from build123d import *

# Parameters (mm, degrees)
BOSS_EXTRUDE1_DEPTH = 2
SKETCH2_R           = 6
CUT_EXTRUDE1_DEPTH  = 124
BOSS_EXTRUDE2_DEPTH = 20


with BuildPart() as part:
    # Sketch1 → Boss-Extrude1 (new body)
    with BuildSketch(Plane.XY):
        Polygon((-55, 0), (55, 0), (20, 110), (-20, 110), align=None)
    extrude(amount=BOSS_EXTRUDE1_DEPTH)

    # Sketch2 → Cut-Extrude1 (cut, through all)
    with BuildSketch(Plane.XY.offset(2)):
        with Locations((0, 90)):
            Circle(SKETCH2_R)
    extrude(amount=-CUT_EXTRUDE1_DEPTH, mode=Mode.SUBTRACT)

    # Sketch4 → Boss-Extrude2 (add)
    with BuildSketch(Plane.XY.offset(2)):
        Polygon((-55, 0), (-54.363636364, 2), (54.363636364, 2), (55, 0), align=None)
    extrude(amount=BOSS_EXTRUDE2_DEPTH)


solid = part.part
Here's how the part is built. I have some questions about the finished solid (model axes, mm). Coordinates: 2 decimals unless noted, no trailing zeros. Order: outer loops, then holes, each group sorted by start corner. A loop starts at its lowest first (then second) coordinate and runs counter-clockwise, first axis right, second up. Notation, with made-up numbers: (0, -39) -> (56, -39) arc R12 ccw to (56, -16) -> close; hole circle Ø10 at (11, -22). An arc over 180 degrees is marked (long way). Answer in a Markdown table with one row per item.
(1) I want a section at B-B on y = 93. List the corners of the cut face in (x, z) for me.
Answer key:
| item | result |
|---|---|
| outline | (-25.41, 0) -> (-5.2, 0) -> (-5.2, 2) -> (-25.41, 2) -> close; (5.2, 0) -> (25.41, 0) -> (25.41, 2) -> (5.2, 2) -> close |
(2) Will these pins go through, and if not, where does the flat tip stop? pin 1 Ø12 at (y, z) = (43.5, 5) entering from +X; pin 2 Ø4 at (x, z) = (18.5, 13) entering from +Y; pin 3 Ø10 at (x, y) = (-38, 61.5) entering from -Z; pin 4 Ø10 at (x, y) = (-18, 48) entering from +Z.
Answer key:
| item | result |
|---|---|
| pin 1 | x = 42.81 |
| pin 2 | y = 2 |
| pin 3 | z = 0 |
| pin 4 | z = 2 |
(3) I want a section at D-D on x = -33. List the corners of the cut face in (y, z) for me.
Answer key:
| item | result |
|---|---|
| outline | (0, 0) -> (69.14, 0) -> (69.14, 2) -> (2, 2) -> (2, 22) -> (0, 22) -> close |
(4) I want a section at C-C on y = 33. List the corners of the cut face in (x, z) for me.
Answer key:
| item | result |
|---|---|
| outline | (-44.5, 0) -> (44.5, 0) -> (44.5, 2) -> (-44.5, 2) -> close |
(5) I want a section at A-A on x = 0. List the corners of the cut face in (y, z) for me.
Answer key:
| item | result |
|---|---|
| outline | (0, 0) -> (84, 0) -> (84, 2) -> (2, 2) -> (2, 22) -> (0, 22) -> close; (96, 0) -> (110, 0) -> (110, 2) -> (96, 2) -> close |
(6) Thinking about a two-plate mould opening in Y: for faces 1 (the face through (1, 0, 11)), 2 (the face through (-1, 45, 2)), 3 (the face through (-0.78, 95.95, 1.01)), 4 (the face through (-1, 2, 12)), which applies, +Y half, -Y half, draft (parallel to the pull), parting line (faces both ways), or undercut?
Answer key:
| item | result |
|---|---|
| face 1 | -Y half |
| face 2 | draft |
| face 3 | undercut |
| face 4 | +Y half |
(7) Please list where these lines run through material, in increasing order: probe 1 along Y at (x, z) = (0, 1.15); probe 2 along Z at (x, y) = (45.5, 17).
Answer key:
| item | result |
|---|---|
| probe 1 | 0 to 84, 96 to 110 |
| probe 2 | 0 to 2 |
